```python
from build123d import *

# Parameters (mm, degrees)
SKETCH1_W           = 169.8
SKETCH1_H           = 167.3
BOSS_EXTRUDE1_DEPTH = 2.4
SKETCH2_R           = 7.5
BOSS_EXTRUDE2_DEPTH = 15
SKETCH6_R           = 15
BOSS_EXTRUDE4_DEPTH = 3
SKETCH7_W           = 5.2
SKETCH7_H           = 2.7
CUT_EXTRUDE1_DEPTH  = 121.537680831
FILLET2_R           = 1.5


with BuildPart() as part:
    # Sketch1 → Boss-Extrude1 (new, symmetric)
    with BuildSketch(Plane(origin=(0, 0, 0), x_dir=(1, 0, 0), z_dir=(0, 1, 0))):
        Rectangle(SKETCH1_W, SKETCH1_H)
    extrude(amount=BOSS_EXTRUDE1_DEPTH, both=True)

    # Sketch2 → Boss-Extrude2 (add)
    with BuildSketch(Plane(origin=(0, 2.4, 0), x_dir=(1, 0, 0), z_dir=(0, 1, 0))):
        with Locations(Location((0, 0, 0), (0, 0, 270))):
            Circle(SKETCH2_R)
    extrude(amount=BOSS_EXTRUDE2_DEPTH)

    # Sketch6 → Boss-Extrude4 (add)
    with BuildSketch(Plane(origin=(0, 17.4, 0), x_dir=(1, 0, 0), z_dir=(0, 1, 0))):
        with Locations(Location((0, 0, 0), (0, 0, 270))):
            Circle(SKETCH6_R)
    extrude(amount=BOSS_EXTRUDE4_DEPTH)

    # Sketch7 → Cut-Extrude1 (cut, through all)
    with BuildSketch(Plane(origin=(0, 2.4, 0), x_dir=(1, 0, 0), z_dir=(0, 1, 0))):
        with Locations((-82.3, -82.3)):
            Rectangle(SKETCH7_W, SKETCH7_H)
        with Locations((82.3, -82.3)):
            Rectangle(SKETCH7_W, SKETCH7_H)
    extrude(amount=-CUT_EXTRUDE1_DEPTH, mode=Mode.SUBTRACT)

    # Fillet2
    fillet2_edges = [part.edges().sort_by_distance(p)[0] for p in [
        (0, 17.4, -15),
        (0, 20.4, -15),
    ]]
    fillet(fillet2_edges, radius=FILLET2_R - 0.0001)  # a hair under: the kernel refuses the full size


solid = part.part
```
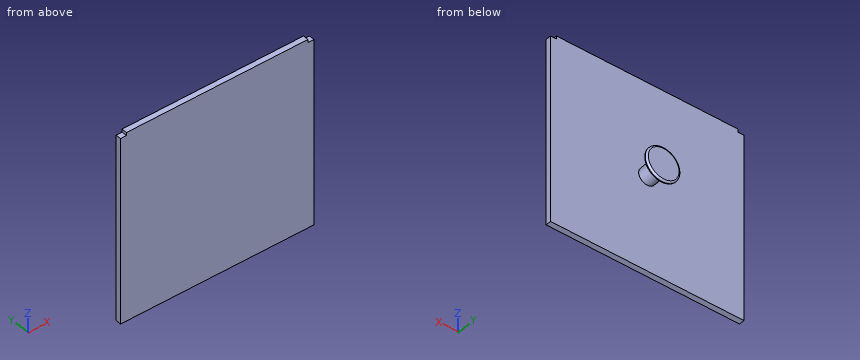
For this review, take the finished solid that the model builds, in its own axes (mm). Give positions to 0.01 mm unless a question says otherwise; leave off trailing zeros. Order: outer loops, then holes, each group sorted by start corner. A loop starts at its lowest first (then second) coordinate and runs counter-clockwise, first axis right, second up.
1) Take a section at C-C (y = 15). Give the boundary of the cut face in (x, z).
2) Wall thickness on line 1 (Y direction, x = 1, z = -11); line 2 (Y direction, x = -43, z = 68); line 3 (X direction, y = 12, z = 0): over which ranges is each line inside the solid? List them lowest first.
3) Take a section at D-D (z = 50). Give the boundary of the cut face in (x, y).
4) Insertion check: pin 1 (3 mm diameter, centred on y = 0.5, z = 82.5, fed in from +X); pin 2 (1.4 mm diameter, centred on x = 83, y = 0.5, fed in from +Z). Each pin has a flat end and moves straight along its axis. Give the tip position at first contact, or say it passes through.
Derived:
1. outline: circle Ø15 at (0, 0)
2. line 1: y = -2.4 to 2.4, 17.4 to 20.4
2. line 2: y = -2.4 to 2.4
2. line 3: x = -7.5 to 7.5
3. outline: (-84.9, -2.4) - (84.9, -2.4) - (84.9, 2.4) - (-84.9, 2.4) - close
4. pin 1: stops at x = 79.7
4. pin 2: stops at z = 80.95
